from build123d import *

# Parameters (mm, degrees)
PAD030_DEPTH    = 1
PAD031_DEPTH    = 3
SKETCH049_R     = 1.6
POCKET019_DEPTH = 5


with BuildPart() as part:
    # Sketch047 → Pad030 (new body)
    with BuildSketch(Plane.XY):
        with BuildLine():
            Line((-55.625, 47.125), (-55.625, -47.125))
            ThreePointArc((-55.625, -47.125), (-55.332107, -47.832107), (-54.625, -48.125))
            Line((-54.625, -48.125), (54.625, -48.125))
            ThreePointArc((54.625, -48.125), (55.332107, -47.832107), (55.625, -47.125))
            Line((55.625, -47.125), (55.625, 47.125))
            ThreePointArc((55.625, 47.125), (55.332107, 47.832107), (54.625, 48.125))
            Line((54.625, 48.125), (-54.625, 48.125))
            ThreePointArc((-54.625, 48.125), (-55.332107, 47.832107), (-55.625, 47.125))
        make_face()
    extrude(amount=PAD030_DEPTH)

    # Sketch048 → Pad031 (join)
    with BuildSketch(Plane.XY):
        with BuildLine():
            Line((-55.625, 47.125), (-55.625, -47.125))
            ThreePointArc((-55.625, -47.125), (-55.332107, -47.832107), (-54.625, -48.125))
            Line((-54.625, -48.125), (54.625, -48.125))
            ThreePointArc((54.625, -48.125), (55.332107, -47.832107), (55.625, -47.125))
            Line((55.625, -47.125), (55.625, 47.125))
            ThreePointArc((55.625, 47.125), (55.332107, 47.832107), (54.625, 48.125))
            Line((54.625, 48.125), (-54.625, 48.125))
            ThreePointArc((-54.625, 48.125), (-55.332107, 47.832107), (-55.625, 47.125))
        make_face()
        with BuildLine():
            Line((-54.625, 46.125), (-54.625, -46.125))
            ThreePointArc((-54.625, -46.125), (-54.332107, -46.832107), (-53.625, -47.125))
            Line((-53.625, -47.125), (53.625, -47.125))
            ThreePointArc((53.625, -47.125), (54.332107, -46.832107), (54.625, -46.125))
            Line((54.625, -46.125), (54.625, 46.125))
            ThreePointArc((54.625, 46.125), (54.332107, 46.832107), (53.625, 47.125))
            Line((53.625, 47.125), (-53.625, 47.125))
            ThreePointArc((-53.625, 47.125), (-54.332107, 46.832107), (-54.625, 46.125))
        make_face(mode=Mode.SUBTRACT)
    extrude(amount=-PAD031_DEPTH)

    # Sketch049 → Pocket019 (cut)
    with BuildSketch(Plane.XY):
        with Locations((-49.5, 40)):
            Circle(SKETCH049_R)
        with Locations((-30, 40)):
            Circle(SKETCH049_R)
        with Locations((30, 40)):
            Circle(SKETCH049_R)
        with Locations((-30, -42)):
            Circle(SKETCH049_R)
        with Locations((-49.5, -42)):
            Circle(SKETCH049_R)
        with Locations((30, -42)):
            Circle(SKETCH049_R)
        with Locations((49.5, -42)):
            Circle(SKETCH049_R)
    extrude(amount=POCKET019_DEPTH, mode=Mode.SUBTRACT)


with BuildPart() as part_1:
    # Body013 placement: moved
    add(part.part.moved(Location((0, 0, 36.1))))


solid = part_1.part
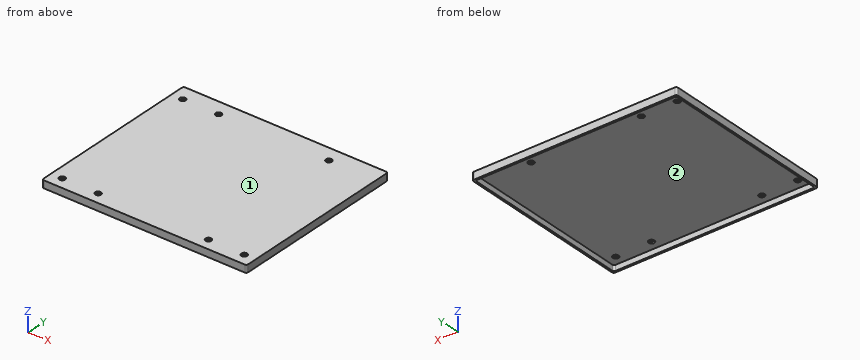
Read the model definition and answer for the solid it produces. Units are mm, in the model's axes. Face numbers are marked on the shaded views. Round coordinates to 2 decimals unless told otherwise and drop trailing zeros. Write each loop counter-clockwise with the first axis right and the second up, starting at its lowest first coordinate (ties: lowest second). Pieces come first, ordered by that corner, then holes. Notation, with made-up numbers: (54.25, -37) - (87.25, -37) arc R18 ccw to (87.25, -4) - close; hole circle Ø3 at (60.25, 33). An arc over 180 degrees is marked (long way). One line per question, with ' | ' between items. Start each with the question number.
1. Section D-D (x = -49.5) is taken. Determine the outline of the cut face in (y, z) (3 decimals).
2. Section B-B (x = 49.5) is taken. Determine the outline of the cut face in (y, z) (3 decimals).
3. Each of these flat-tipped pins is pushed along its axis until it touches: pin 1 (4 mm diameter, centred on x = -30, y = -42, fed in from -Z); pin 2 (2.5 mm diameter, centred on x = 49.5, y = -42, fed in from +Z). Where does it stop, or does it pass through?
4. Section A-A (y = -42) is taken. Determine the outline of the cut face in (x, z) (3 decimals), and give its area (3 significant figures).
5. For a pull along X with two mould halves and no side action, classify the marked faces 1 and 2 as +X half, -X half, draft (parallel to the pull), parting line (faces both ways), or undercut.
6. Find the intervals of material crossed by probe 1 along X at (y, z) = (-42, 36.7) (3 decimals); probe 2 along Y at (x, z) = (30, 36.5) (3 decimals); probe 3 along X at (y, z) = (22, 34.15) (3 decimals), in increasing order. Write a range as [from, to].
7. Section C-C (z = 34.6) is taken. Determine the outline of the cut face in (x, y) (3 decimals).
Filled in:
1) outline: (-48.125, 33.1) - (-47.125, 33.1) - (-47.125, 36.1) - (-43.6, 36.1) - (-43.6, 37.1) - (-48.125, 37.1) - close; (-40.4, 36.1) - (38.4, 36.1) - (38.4, 37.1) - (-40.4, 37.1) - close; (41.6, 36.1) - (47.125, 36.1) - (47.125, 33.1) - (48.125, 33.1) - (48.125, 37.1) - (41.6, 37.1) - close
2) outline: (-48.125, 33.1) - (-47.125, 33.1) - (-47.125, 36.1) - (-43.6, 36.1) - (-43.6, 37.1) - (-48.125, 37.1) - close; (-40.4, 36.1) - (47.125, 36.1) - (47.125, 33.1) - (48.125, 33.1) - (48.125, 37.1) - (-40.4, 37.1) - close
3) pin 1: z = 36.1 | pin 2: through
4) outline: (-55.625, 33.1) - (-54.625, 33.1) - (-54.625, 36.1) - (-51.1, 36.1) - (-51.1, 37.1) - (-55.625, 37.1) - close; (-47.9, 36.1) - (-31.6, 36.1) - (-31.6, 37.1) - (-47.9, 37.1) - close; (-28.4, 36.1) - (28.4, 36.1) - (28.4, 37.1) - (-28.4, 37.1) - close; (31.6, 36.1) - (47.9, 36.1) - (47.9, 37.1) - (31.6, 37.1) - close; (51.1, 36.1) - (54.625, 36.1) - (54.625, 33.1) - (55.625, 33.1) - (55.625, 37.1) - (51.1, 37.1) - close | area: 104 mm²
5) face 1: draft | face 2: undercut
6) probe 1: [-55.625, -51.1], [-47.9, -31.6], [-28.4, 28.4], [31.6, 47.9], [51.1, 55.625] | probe 2: [-48.125, -43.6], [-40.4, 38.4], [41.6, 48.125] | probe 3: [-55.625, -54.625], [54.625, 55.625]
7) outline: (-55.625, -47.125) arc R1 ccw to (-54.625, -48.125) - (54.625, -48.125) arc R1 ccw to (55.625, -47.125) - (55.625, 47.125) arc R1 ccw to (54.625, 48.125) - (-54.625, 48.125) arc R1 ccw to (-55.625, 47.125) - close; hole (-54.625, -46.125) arc R1 ccw to (-53.625, -47.125) - (53.625, -47.125) arc R1 ccw to (54.625, -46.125) - (54.625, 46.125) arc R1 ccw to (53.625, 47.125) - (-53.625, 47.125) arc R1 ccw to (-54.625, 46.125) - close
